The model under review builds one solid part; all positions refer to its coordinate system, in mm. A direction names the side the tool comes from. Round coordinates to 2 decimals unless told otherwise and drop trailing zeros. Write each loop counter-clockwise with the first axis right and the second up, starting at its lowest first coordinate (ties: lowest second). Pieces come first, ordered by that corner, then holes. Notation, with made-up numbers: (4, -3) - (26, -3) arc R35 cw to (26, 36) - close; hole circle Ø3 at (0.5, 7.5). An arc over 180 degrees is marked (long way). One line per question, with ' | ' between items. Start each with the question number.
```python
from build123d import *

# Parameters (mm, degrees)
SKETCH1_W           = 116
SKETCH1_H           = 96
BOSS_EXTRUDE1_DEPTH = 6
SKETCH2_W           = 116
SKETCH2_H           = 96
SKETCH2_W_2         = 110
SKETCH2_H_2         = 90
BOSS_EXTRUDE2_DEPTH = 35
SKETCH3_W           = 71.6
SKETCH3_H           = 24.5
SKETCH3_W_2         = 13.5
SKETCH3_H_2         = 16.8
CUT_EXTRUDE1_DEPTH  = 35
SKETCH4_W           = 5
SKETCH4_H           = 18
CUT_EXTRUDE2_DEPTH  = 4
SKETCH6_R           = 3.75
CUT_EXTRUDE3_DEPTH  = 3
SKETCH7_W           = 110
SKETCH7_H           = 90
SKETCH7_W_2         = 80.6
SKETCH7_H_2         = 28.5
SKETCH7_W_3         = 17.5
SKETCH7_H_3         = 20.8
CUT_EXTRUDE4_DEPTH  = 4
SKETCH8_W           = 7
SKETCH8_H           = 35
SKETCH8_W_2         = 15
SKETCH8_H_2         = 6
SKETCH8_W_3         = 25
BOSS_EXTRUDE3_DEPTH = 9
CUT_EXTRUDE6_START  = -1
CUT_EXTRUDE6_DEPTH  = 114


with BuildPart() as part:
    # Sketch1 → Boss-Extrude1 (new body)
    with BuildSketch(Plane(origin=(0, 0, 0), x_dir=(1, 0, 0), z_dir=(0, 1, 0))):
        Rectangle(SKETCH1_W, SKETCH1_H)
    extrude(amount=BOSS_EXTRUDE1_DEPTH)

    # Sketch2 → Boss-Extrude2 (add)
    with BuildSketch(Plane(origin=(0, 6, 0), x_dir=(1, 0, 0), z_dir=(0, 1, 0))):
        Rectangle(SKETCH2_W, SKETCH2_H)
        Rectangle(SKETCH2_W_2, SKETCH2_H_2, mode=Mode.SUBTRACT)
    extrude(amount=BOSS_EXTRUDE2_DEPTH)

    # Sketch3 → Cut-Extrude1 (cut)
    with BuildSketch(Plane(origin=(0, 6, 0), x_dir=(1, 0, 0), z_dir=(0, 1, 0))):
        with Locations((10.2, -22.75)):
            Rectangle(SKETCH3_W, SKETCH3_H)
        with Locations((-34.35, 20.9)):
            Rectangle(SKETCH3_W_2, SKETCH3_H_2)
    extrude(amount=-CUT_EXTRUDE1_DEPTH, mode=Mode.SUBTRACT)

    # Sketch4 → Cut-Extrude2 (cut)
    with BuildSketch(Plane(origin=(0, 6, 0), x_dir=(1, 0, 0), z_dir=(0, 1, 0))):
        with Locations((-28.1, -22.75)):
            Rectangle(SKETCH4_W, SKETCH4_H)
    extrude(amount=-CUT_EXTRUDE2_DEPTH, mode=Mode.SUBTRACT)

    # Sketch6 → Cut-Extrude3 (cut)
    with BuildSketch(Plane(origin=(58, 0, 0), x_dir=(0, 0, -1), z_dir=(1, 0, 0))):
        with Locations((-35, 27.500245912)):
            Circle(SKETCH6_R)
        with BuildLine():
            Line((17.5, 12), (25.5, 12))
            ThreePointArc((25.5, 12), (29.5, 8), (25.5, 4))
            Line((25.5, 4), (17.5, 4))
            ThreePointArc((17.5, 4), (13.5, 8), (17.5, 12))
        make_face()
    extrude(amount=-CUT_EXTRUDE3_DEPTH, mode=Mode.SUBTRACT)

    # Sketch7 → Cut-Extrude4 (cut)
    with BuildSketch(Plane(origin=(0, 6, 0), x_dir=(1, 0, 0), z_dir=(0, 1, 0))):
        Rectangle(SKETCH7_W, SKETCH7_H)
        with Locations((7.7, -22.75)):
            Rectangle(SKETCH7_W_2, SKETCH7_H_2, mode=Mode.SUBTRACT)
        with Locations((-34.35, 20.9)):
            Rectangle(SKETCH7_W_3, SKETCH7_H_3, mode=Mode.SUBTRACT)
    extrude(amount=-CUT_EXTRUDE4_DEPTH, mode=Mode.SUBTRACT)

    # Sketch8 → Boss-Extrude3 (add)
    with BuildSketch(Plane(origin=(0, 2, 0), x_dir=(1, 0, 0), z_dir=(0, 1, 0))):
        with Locations((-51.5, -27.5)):
            Rectangle(SKETCH8_W, SKETCH8_H)
        with Locations((47.5, 42)):
            Rectangle(SKETCH8_W_2, SKETCH8_H_2)
        with Locations((-42.5, 42)):
            Rectangle(SKETCH8_W_3, SKETCH8_H_2)
    extrude(amount=BOSS_EXTRUDE3_DEPTH)

    # Sketch10 → Cut-Extrude6 (cut)
    with BuildSketch(Plane(origin=(58, 0, 0), x_dir=(0, 0, -1), z_dir=(1, 0, 0)).offset(CUT_EXTRUDE6_START)):
        Polygon((-32, 41), (-32, 35.5), (-37.5, 35.5), (-37.5, 37.5), (-34, 37.5), (-34, 41), align=None)
        Polygon((36, 41), (38, 41), (38, 35.5), (32.5, 35.5), (32.5, 37.5), (36, 37.5), align=None)
    extrude(amount=-CUT_EXTRUDE6_DEPTH, mode=Mode.SUBTRACT)


solid = part.part
```
1. Clearance check with flat-ended pins moving along their axes: P1, Ø1, axis at x = -19.5, z = 0, coming from the +Y side; P2, Ø5, axis at x = 45.5, z = -41, coming from the +Y side. State where each tip first meets the part, or that it passes through.
2. Add section A-A, the plane x = 24.5. Write out the cut boundary in (y, z), then the cut area to 3 significant figures.
3. Add section B-B, the plane y = 18. Write out the cut boundary in (x, z).
4. The part is to be moulded in two halves that separate along Z. For faces 1 (the face through (-1, 0, -1)), 2 (the face through (-32.6, 4, 23)), 3 (the face through (-1, 20, -48)), say which applies: pulls with the +Z half, pulls with the -Z half, needs draft (parallel to the pull), parting line crosses it, or undercut.
5. Machinability: for faces 4 (the face through (-57, 37, -36)), 5 (the face through (-34, 3, -12.5)), 6 (the face through (56.521, 27.665, 38.746)), 7 (the face through (48, 4, 23)), which of the approach directions +Z, -Z, +X, -X, +Y, -Y give a long, thin tool a straight path to every point of the face, cutting with its end or side? Answer none if there is none.
6. Add section C-C, the plane z = 40.5. Write out the cut boundary in (x, y), then the cut area to 3 significant figures.
7. Add section D-D, the plane y = 8. Write out the cut boundary in (x, z).
8. Wall thickness on line 1 along Y through (x, z) = (56, 35); line 2 along X through (y, z) = (36, 2.5); line 3 along Z through (x, y) = (22, 33): over which ranges is each line inside the solid? List them lowest first. Write a range as [from, to].
Geometry check:
1) P1: stops at y = 2 | P2: stops at y = 11
2) outline: (0, -48) - (41, -48) - (41, -45) - (2, -45) - (2, 8.5) - (6, 8.5) - (6, 10.5) - (0, 10.5) - close; (0, 35) - (6, 35) - (6, 37) - (2, 37) - (2, 45) - (41, 45) - (41, 48) - (0, 48) - close | area: 393 mm2
3) outline: (-58, -48) - (58, -48) - (58, 48) - (-58, 48) - close; hole (-55, -45) - (55, -45) - (55, 45) - (-55, 45) - close
4) face 1: needs draft | face 2: undercut | face 3: pulls with the -Z half
5) face 4: none | face 5: +Y, -Y | face 6: +X | face 7: +Y
6) outline: (-58, 0) - (58, 0) - (58, 41) - (55, 41) - (55, 2) - (-48, 2) - (-48, 11) - (-55, 11) - (-55, 41) - (-58, 41) - close | area: 529 mm2
7) outline: (-58, -48) - (58, -48) - (58, -29.5) - (55, -29.5) - (55, -39) - (40, -39) - (40, -45) - (-30, -45) - (-30, -39) - (-55, -39) - (-55, 10) - (-48, 10) - (-48, 45) - (55, 45) - (55, -13.5) - (58, -13.5) - (58, 48) - (-58, 48) - close
8) line 1: y = [0, 23.75], [31.25, 35.5], [37.5, 41] | line 2: x = [-58, -55], [55, 58] | line 3: z = [-48, -45], [45, 48]
